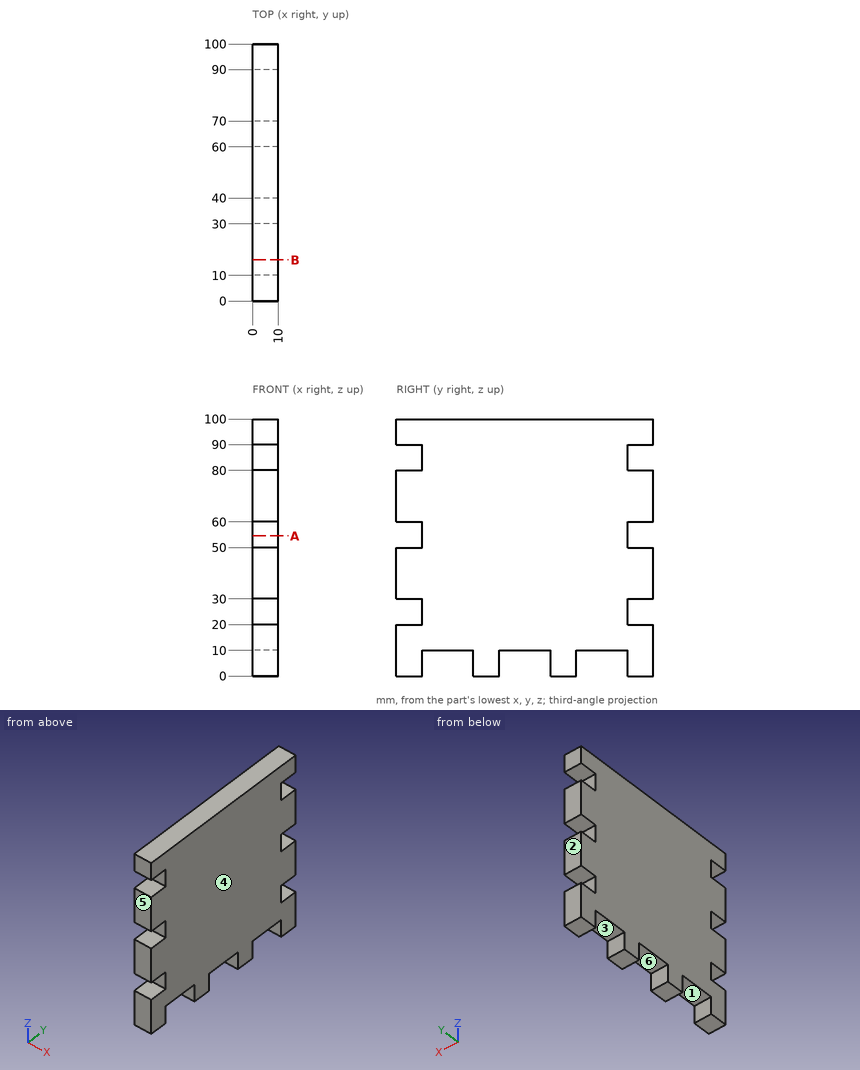
Verification items for this drawing (mm, ordinates from the low corner). A direction names the side the tool comes from. Coordinates: 2 decimals unless noted, no trailing zeros. Order: outer loops, then holes, each group sorted by start corner. A loop starts at its lowest first (then second) coordinate and runs counter-clockwise, first axis right, second up.
Q1. Sectioned sample at A-A on z = 54.5. Record the cut outline in (x, y).
Reply:
outline: (0, 10) - (10, 10) - (10, 90) - (0, 90) - close
Q2. Tool access check on the marked faces 5 and 6. Record the directions out of +Z, -Z, +X, -X, +Y, -Y that give a thin tool (end or side, any length) a straight path to the whole face; none if there is none.
Reply:
face 5: +Z, -Z, +X, -X, -Y
face 6: -Z, +X, -X
Q3. Sectioned sample at B-B on y = 16. Record the cut outline in (x, z), and give its area (3 significant figures).
Reply:
outline: (0, 10) - (10, 10) - (10, 100) - (0, 100) - close
area: 900 mm2
Q4. Thickness scan on probe 1 along Y at (x, z) = (9.5, 7); probe 2 along Z at (x, y) = (4.5, 46.5); probe 3 along Y at (x, z) = (6.75, 83). Record the ranges inside material, lowest first.
Reply:
probe 1: y = 0 to 10, 30 to 40, 60 to 70, 90 to 100
probe 2: z = 10 to 100
probe 3: y = 10 to 90
Q5. Draft check along Y on the marked faces 1, 2, 3 and 4. Enter one of: released by +Y, released by -Y, zero draft, split by the parting line, or undercut.
Reply:
face 1: undercut
face 2: released by +Y
face 3: undercut
face 4: zero draft
Q6. Depth check by flat-ended pin: pin 1 Ø6 at (x, y) = (7.5, 48.5) entering from -Z. Enter the tip coordinate at first touch or a pass-through.
Reply:
pin 1: stops at z = 10
